Verification items for the finished model (mm, model axes). A direction names the side the tool comes from. Coordinates: 2 decimals unless noted, no trailing zeros. Loops run counter-clockwise (first coordinate to the right, second up) from the corner with the lowest first, then second, coordinate; pieces in that order, holes last. Notation, with made-up numbers: (29, 53.5) -> (67, 53.5) arc R16 cw to (67, 57.5) -> close; hole circle Ø2 at (7.25, -11). An arc over 180 degrees is marked (long way). Write item = value, one per line.
```python
from build123d import *

# Parameters (mm, degrees)
SKETCH2_W               = 8.4
SKETCH2_H               = 10
BOSS_EXTRUDE1_DEPTH     = 11.3
SKETCH5_W               = 8.4
SKETCH5_H               = 1.5
CUT_EXTRUDE2_DEPTH      = 11.3
SKETCH7_W               = 1.6
SKETCH7_H               = 3.3
CUT_EXTRUDE4_DEPTH      = 8.4
SKETCH9_W               = 8.4
SKETCH9_H               = 1.7
CUT_EXTRUDE5_DEPTH      = 6.8
SKETCH12_W              = 6.8
SKETCH12_H              = 1.6
BOSS_EXTRUDE3_DEPTH     = 1.6
FILLET1_R               = 1
M3_5X0_6_TAPPED_HOLE1_D = 2.9
SKETCH20_W              = 1.6
SKETCH20_H              = 1.6
CUT_EXTRUDE6_DEPTH      = 6.8


with BuildPart() as part:
    # Sketch2 → Boss-Extrude1 (new body)
    with BuildSketch(Plane(origin=(0, 0, 0), x_dir=(1, 0, 0), z_dir=(0, 1, 0))):
        Rectangle(SKETCH2_W, SKETCH2_H)
    extrude(amount=BOSS_EXTRUDE1_DEPTH)

    # Sketch5 → Cut-Extrude2 (cut)
    with BuildSketch(Plane(origin=(4.2, 0, 0), x_dir=(0, 0, -1), z_dir=(1, 0, 0))):
        with Locations((0.8, 10.55)):
            Rectangle(SKETCH5_W, SKETCH5_H)
    extrude(amount=-CUT_EXTRUDE2_DEPTH, mode=Mode.SUBTRACT)

    # Sketch7 → Cut-Extrude4 (cut)
    with BuildSketch(Plane(origin=(0, 0, -5), x_dir=(-1, 0, 0), z_dir=(0, 0, -1))):
        with Locations((-3.4, 8.15)):
            Rectangle(SKETCH7_W, SKETCH7_H)
    extrude(amount=-CUT_EXTRUDE4_DEPTH, mode=Mode.SUBTRACT)

    # Sketch9 → Cut-Extrude5 (cut)
    with BuildSketch(Plane(origin=(2.6, 0, 0), x_dir=(0, 0, -1), z_dir=(1, 0, 0))):
        with Locations((0.8, 8.95)):
            Rectangle(SKETCH9_W, SKETCH9_H)
    extrude(amount=-CUT_EXTRUDE5_DEPTH, mode=Mode.SUBTRACT)

    # Sketch12 → Boss-Extrude3 (add)
    with BuildSketch(Plane(origin=(0, 0, 3.4), x_dir=(-1, 0, 0), z_dir=(0, 0, -1))):
        with Locations((0.8, 8.9)):
            Rectangle(SKETCH12_W, SKETCH12_H)
    extrude(amount=BOSS_EXTRUDE3_DEPTH)

    # Fillet1
    fillet1_edges = [part.edges().sort_by_distance(p)[0] for p in [
        (4.2, 3.25, -5),
        (0, 0, 5),
        (0, 0, -5),
        (4.2, 0, 0),
        (4.2, 5.65, 5),
    ]]
    fillet(fillet1_edges, radius=FILLET1_R)

    # M3.5x0.6 Tapped Hole1 (through all)
    with Locations(Plane(origin=(0, 0, 0), x_dir=(-1, 0, 0), z_dir=(0, -1, 0))):
        with Locations((1.3, -0.5)):
            Hole(M3_5X0_6_TAPPED_HOLE1_D / 2)

    # Sketch20 → Cut-Extrude6 (cut)
    with BuildSketch(Plane(origin=(2.6, 0, 0), x_dir=(0, 0, -1), z_dir=(1, 0, 0))):
        with Locations((-2.6, 8.9)):
            Rectangle(SKETCH20_W, SKETCH20_H)
    extrude(amount=-CUT_EXTRUDE6_DEPTH, mode=Mode.SUBTRACT)


solid = part.part
```
1) Sectioned sample at A-A, the plane z = 0.5. Record the cut outline in (x, y).
Ans:
outline = (-4.2, 0) -> (-2.75, 0) -> (-2.75, 8.1) -> (-4.2, 8.1) -> close; (0.15, 0) -> (3.2, 0) arc R1 ccw to (4.2, 1) -> (4.2, 6.5) -> (2.6, 6.5) -> (2.6, 8.1) -> (0.15, 8.1) -> close
2) Depth check by flat-ended pin: pin 1 Ø0.5 at (x, z) = (3.5, 0) entering from +Y. Enter the tip coordinate at first touch or a pass-through.
Ans:
pin_1 = 6.5
3) Material ranges on line 1 (Z direction, x = -1.3, y = 6.5); line 2 (Y direction, x = -3, z = 0.25); line 3 (Z direction, x = -0.75, y = 2.5), recorded low to high.
Ans:
line_1 = -5 to -0.95, 1.95 to 5
line_2 = 0 to 8.1
line_3 = -5 to -0.84, 1.84 to 5
4) Release check for a two-part mould opening along Z. For faces 4 (the face through (-2.75, 4.11, 0.44)), 5 (the face through (2.6, 7, -1)), 6 (the face through (3.915, 3.788, -4.699)) record: pulls with the +Z half, pulls with the -Z half, needs draft (parallel to the pull), parting line crosses it, or undercut.
Ans:
face_4 = undercut
face_5 = needs draft
face_6 = pulls with the -Z half
5) Sectioned sample at D-D, the plane z = -2.25. Record the cut outline in (x, y).
Ans:
outline = (-4.2, 0) -> (3.2, 0) arc R1 ccw to (4.2, 1) -> (4.2, 6.5) -> (2.6, 6.5) -> (2.6, 8.1) -> (-4.2, 8.1) -> close
6) Sectioned sample at C-C, the plane y = 4.75. Record the cut outline in (x, z), plus the area to 3 significant figures.
Ans:
outline = (-4.2, -5) -> (3.2, -5) arc R1 ccw to (4.2, -4) -> (4.2, 4) arc R1 ccw to (3.2, 5) -> (-4.2, 5) -> close; hole circle Ø2.9 at (-1.3, 0.5)
area = 77.0 mm2
7) Tool access check on faces 1 (the face through (-1, 5, -5)), 2 (the face through (3, 6.5, -1)), 3 (the face through (0, 8.1, -1)). Record the directions out of +Z, -Z, +X, -X, +Y, -Y that give a thin tool (end or side, any length) a straight path to the whole face; none if there is none.
Ans:
face_1 = -Z, +X, -X, +Y, -Y
face_2 = -Z, +X, +Y
face_3 = -Z, +X, -X, +Y
8) Sectioned sample at B-B, the plane x = -1.3. Record the cut outline in (y, z), plus the area to 3 significant figures.
Ans:
outline = (0, -4) arc R1 ccw to (1, -5) -> (8.1, -5) -> (8.1, -0.95) -> (0, -0.95) -> close; (0, 1.95) -> (8.1, 1.95) -> (8.1, 3.4) -> (11.3, 3.4) -> (11.3, 5) -> (1, 5) arc R1 ccw to (0, 4) -> close
area = 62.2 mm2
